Design review of the part built by this model. Coordinates are the model's own, in mm. A direction names the side the tool comes from. Coordinates: 2 decimals unless noted, no trailing zeros. Loops run counter-clockwise (first coordinate to the right, second up) from the corner with the lowest first, then second, coordinate; pieces in that order, holes last. Notation, with made-up numbers: (51.25, 80.25) - (91.25, 80.25) arc R17 cw to (91.25, 93.25) - close; hole circle Ø11 at (-16, 20). An arc over 180 degrees is marked (long way). Return JSON: item names as keys, results as strings. Group by question number.
from build123d import *

# Parameters (mm, degrees)
SKETCH_1_W           = 175
SKETCH_1_H           = 160
EXTRUDE_1_DEPTH      = 193
FILLET_8_R           = 40
SHELL_2_T            = -5
SKETCH_9_W           = 95
SKETCH_9_H           = 80
CUT_EXTRUDE_3_DEPTH  = 10
SKETCH_10_R          = 35
CUT_EXTRUDE_4_DEPTH  = 160
SKETCH_12_W          = 40
SKETCH_12_H          = 60
CUT_EXTRUDE_5_DEPTH  = 20
CUT_EXTRUDE_6_DEPTH  = 80
SKETCH_15_R          = 2.5
CUT_EXTRUDE_8_DEPTH  = 5
SKETCH_17_R          = 2.5
SKETCH_17_W          = 20
SKETCH_17_H          = 20
CUT_EXTRUDE_10_DEPTH = 5
CUT_EXTRUDE_11_DEPTH = 2
SKETCH_20_R          = 2.5
CUT_EXTRUDE_13_DEPTH = 5


with BuildPart() as part:
    # 草圖1 → 填料-伸長1 (new body)
    with BuildSketch(Plane.XY):
        Rectangle(SKETCH_1_W, SKETCH_1_H)
    extrude(amount=EXTRUDE_1_DEPTH)

    # 圓角8
    fillet_8_edges = [part.edges().sort_by_distance(p)[0] for p in [
        (-87.5, 0, 193),
        (0, -80, 193),
        (87.5, 0, 193),
        (0, 80, 193),
    ]]
    fillet(fillet_8_edges, radius=FILLET_8_R)

    # 薄殼2
    shell_2_openings = [part.faces().sort_by_distance(p)[0] for p in [
        (0, 0, 0),
    ]]
    offset(amount=SHELL_2_T, openings=shell_2_openings)

    # 草圖9 → 除料-伸長3 (cut)
    with BuildSketch(Plane.XY.offset(193)):
        Rectangle(SKETCH_9_W, SKETCH_9_H)
    extrude(amount=-CUT_EXTRUDE_3_DEPTH, mode=Mode.SUBTRACT)

    # 草圖10 → 除料-伸長4 (cut)
    with BuildSketch(Plane(origin=(0, 80, 0), x_dir=(1, 0, 0), z_dir=(0, 1, 0))):
        with Locations((-18.75, -12.103072957)):
            Circle(SKETCH_10_R)
    extrude(amount=-CUT_EXTRUDE_4_DEPTH, mode=Mode.SUBTRACT)

    # 草圖12 → 除料-伸長5 (cut)
    with BuildSketch(Plane(origin=(90, 0, 0), x_dir=(0, 0, -1), z_dir=(1, 0, 0))):
        with Locations((-155.457670656, 0)):
            Rectangle(SKETCH_12_W, SKETCH_12_H)
    extrude(amount=-CUT_EXTRUDE_5_DEPTH, mode=Mode.SUBTRACT)

    # 草圖4 → 除料-伸長6 (cut)
    with BuildSketch(Plane(origin=(0, 0, 0), x_dir=(1, 0, 0), z_dir=(0, 1, 0))):
        Polygon((0, -200), (-165, -200), (-165, 0), (110, 0), (110, -200), align=None)
    extrude(amount=CUT_EXTRUDE_6_DEPTH, mode=Mode.SUBTRACT)

    # 草圖15 → 除料-伸長8 (cut)
    with BuildSketch(Plane(origin=(0, -80, 0), x_dir=(1, 0, 0), z_dir=(0, 1, 0))):
        with Locations(Location((-7.5, -85, 0), (0, 0, 270))):
            Circle(SKETCH_15_R)
        with Locations(Location((7.5, -85, 0), (0, 0, 270))):
            Circle(SKETCH_15_R)
    extrude(amount=CUT_EXTRUDE_8_DEPTH, mode=Mode.SUBTRACT)

    # 草圖17 → 除料-伸長10 (cut)
    with BuildSketch(Plane.ZY.offset(87.5)):
        with Locations((130, -35)):
            Circle(SKETCH_17_R)
        with Locations((142.5, -35)):
            Circle(SKETCH_17_R)
        with Locations((70, -25)):
            Circle(SKETCH_17_R)
        with Locations((95, -25)):
            Circle(SKETCH_17_R)
        with Locations((75, -10)):
            Rectangle(SKETCH_17_W, SKETCH_17_H)
    extrude(amount=-CUT_EXTRUDE_10_DEPTH, mode=Mode.SUBTRACT)

    # 草圖18 → 除料-伸長11 (cut)
    with BuildSketch(Plane(origin=(87.5, 0, 0), x_dir=(0, 0, -1), z_dir=(1, 0, 0))):
        with BuildLine():
            Line((-89.728835328, 0), (-67.728835328, 0))
            ThreePointArc((-67.728835328, 0), (-62.3717018, -23.697451199), (-43.97726554, -39.569211896))
            ThreePointArc((-43.97726554, -39.569211896), (-72.150234213, -32.803686073), (-89.728835328, -9.771506706))
            Line((-89.728835328, -9.771506706), (-89.893994181, -4.771506706))
            Line((-89.893994181, -4.771506706), (-89.728835328, 0))
        make_face()
    extrude(amount=-CUT_EXTRUDE_11_DEPTH, mode=Mode.SUBTRACT)

    # 草圖20 → 除料-伸長13 (cut)
    with BuildSketch(Plane(origin=(85.5, 0, 0), x_dir=(0, 0, -1), z_dir=(1, 0, 0))):
        with Locations((-85.811414754, -7.139379624)):
            Circle(SKETCH_20_R)
    extrude(amount=-CUT_EXTRUDE_13_DEPTH, mode=Mode.SUBTRACT)


solid = part.part
Item 1: Add section C-C (z = 165). State the section outline as (x, y) points, then the cut area to 3 significant figures.
Item 2: Add section A-A (z = 142.5). State the section outline as (x, y) points.
Item 3: Add section B-B (x = 7.5). State the section outline as (y, z) points, then the cut area to 3 significant figures.
Item 4: For faces 4 (the face through (-85, -10, 85)), 5 (the face through (47.5, -20, 191)), 6 (the face through (84, -30, 156)), 7 (the face through (-72.519, -28.642, 177.475)), 8 (the face through (78, -15, 175.458)), list the 3-axis set-ups (+Z, -Z, +X, -X, +Y, -Y) from which the entire face can be reached by the end or side of a thin tool; tool diameter is ignored.
Item 5: Add section D-D (x = -18.75). State the section outline as (y, z) points, then the cut area to 3 significant figures.
Item 6: To check wall thickness, follow line 1 (X direction, y = -78, z = 85); line 2 (X direction, y = -34, z = 87); line 3 (Y direction, x = -84, z = 70). State the ranges of each line that lie inside material, in increasing order. Write a range as from..to.
Item 7: Draft analysis for pull direction Z (two halves, no side actions). For faces 1 (the face through (85, 0, 67)), 2 (the face through (76.094, -39.44, 180.972)), 3 (the face through (-85.035, -34.249, 144.885)), state which applies: pulls with the +Z half, pulls with the -Z half, needs draft (parallel to the pull), parting line crosses it, or undercut.
Item 8: For P1, Ø6, axis at x = -7.5, z = 85, coming from the +Y side; P2, Ø2.5, axis at y = -16, z = 190.5, coming from the -X side; P3, Ø6, axis at x = -23, y = -54.5, coming from the -Z side, all flat-tipped, find the tip position at first contact; note any pin that passes through.
Answers below:
{
 "1": {"outline": "(-85.66, -78.16) - (85.66, -78.16) - (85.66, -30) - (80.38, -30) - (80.38, -72.88) - (-80.38, -72.88) - (-80.38, 0) - (-85.66, 0) - close", "area": "1,520 mm^2"},
 "2": {"outline": "(-87.5, -80) - (87.5, -80) - (87.5, -30) - (82.5, -30) - (82.5, -75) - (-82.5, -75) - (-82.5, -37.5) - (-87.5, -37.5) - close; (-87.5, -32.5) - (-82.5, -32.5) - (-82.5, 0) - (-87.5, 0) - close"},
 "3": {"outline": "(-80, 35.25) - (-75, 35.25) - (-75, 82.5) - (-80, 82.5) - close; (-80, 87.5) - (-75, 87.5) - (-75, 153) arc R35 cw to (-40, 188) - (-40, 193) arc R40 ccw to (-80, 153) - close", "area": "858 mm^2"},
 "4": {"face 4": "-X, +Y", "face 5": "+Z, -Z, +Y", "face 6": "+X, +Y", "face 7": "-Z, +Y", "face 8": "-Z, +X, +Y"},
 "5": {"outline": "(-80, 47.1) - (-75, 47.1) - (-75, 153) arc R35 cw to (-40, 188) - (-40, 193) arc R40 ccw to (-80, 153) - close", "area": "824 mm^2"},
 "6": {"line 1": "x = -87.5..-10, -5..5, 10..87.5", "line 2": "x = -87.5..-82.5, 82.5..87.5", "line 3": "y = -80..-27.5, -22.5..-20"},
 "7": {"face 1": "needs draft", "face 2": "pulls with the +Z half", "face 3": "undercut"},
 "8": {"P1": "stops at y = -75", "P2": "stops at x = -64.41", "P3": "stops at z = 183.31"}
}
